Design review of the part built by this model. Coordinates are the model's own, in mm. Face numbers are marked on the shaded views. A direction names the side the tool comes from. Coordinates: 2 decimals unless noted, no trailing zeros. Write each loop counter-clockwise with the first axis right and the second up, starting at its lowest first coordinate (ties: lowest second). Pieces come first, ordered by that corner, then holes. Notation, with made-up numbers: (55.25, 60.5) - (85.25, 60.5) arc R15 cw to (85.25, 65.5) - close; hole circle Ø4 at (-6.5, 75.5). An arc over 180 degrees is marked (long way). Answer as CSV lines item,"result". Start each with the question number.
Q1. We need section B-B (x = 0). Write out the cut boundary in (y, z).
Q2. Mouldability with a two-part tool opening along X and no side actions: class the marked faces 3, 4 and 5 as pulls with the +X half, pulls with the -X half, needs draft (parallel to the pull), parting line crosses it, or undercut.
Q3. For line 1 along Z through (x, y) = (15, 17); line 2 along Z through (x, y) = (-4, 3); line 3 along X through (y, z) = (0, 27), list the stretches that pass through material, from the lowest coordinate up. Write a range as [from, to].
Q4. We need section C-C (z = 52). Write out the cut boundary in (x, y), plus the area to 3 significant figures.
Q5. Clearance check with flat-ended pins moving along their axes: pin 1 (10 mm diameter, centred on x = 7.5, y = 1, fed in from +Z); pin 2 (3 mm diameter, centred on x = 5.5, z = 44.5, fed in from -Y); pin 3 (5 mm diameter, centred on y = -0.5, z = 52.5, fed in from +X); pin 4 (3 mm diameter, centred on y = -0.5, z = 16.5, fed in from -X). State where each tip first meets the part, or that it passes through.
Q6. Machinability: for the marked faces 1 and 2, which of the approach directions +Z, -Z, +X, -X, +Y, -Y give a long, thin tool a straight path to every point of the face, cutting with its end or side? Answer none if there is none.
Q7. We need section A-A (y = 0). Write out the cut boundary in (x, z).
Q8. We need section D-D (z = 33). Write out the cut boundary in (x, y), plus the area to 3 significant figures.
from build123d import *

# Parameters (mm, degrees)
SKETCH1_R               = 7.5
BOSS_EXTRUDE1_DEPTH     = 56
SKETCH2_W               = 10
SKETCH2_H               = 16
CUT_EXTRUDE1_DEPTH      = 10
CUT_EXTRUDE4_DEPTH      = 57.995613866
CUT_EXTRUDE4_DEPTH_BACK = 57.995613866
CUT_EXTRUDE5_DEPTH      = 57.995613991
CUT_EXTRUDE5_DEPTH_BACK = 57.995613991
SKETCH4_R               = 1.5
FILLET1_R               = 0.1
SKETCH5_W               = 40
SKETCH5_H               = 40
BOSS_EXTRUDE2_DEPTH     = 5


with BuildPart() as part:
    # Sketch1 → Boss-Extrude1 (new body)
    with BuildSketch(Plane.XY):
        Circle(SKETCH1_R)
    extrude(amount=BOSS_EXTRUDE1_DEPTH)

    # Sketch2 → Cut-Extrude1 (cut)
    with BuildSketch(Plane.XY.offset(56)):
        Rectangle(SKETCH2_W, SKETCH2_H)
    extrude(amount=-CUT_EXTRUDE1_DEPTH, mode=Mode.SUBTRACT)

    # Sketch3 → Cut-Extrude4 (cut, two sides: drawn at the far end of the back side and taken through both)
    with BuildSketch(Plane(origin=(0, 0, 0), x_dir=(0, 0, -1), z_dir=(1, 0, 0)).offset(-CUT_EXTRUDE4_DEPTH_BACK)):
        with BuildLine():
            Line((-46, -114.267763227), (-46, -7.5))
            Line((-46, -7.5), (-46, -5.590169944))
            Line((-46, -5.590169944), (-52.952744721, -3.885047998))
            ThreePointArc((-52.952744721, -3.885047998), (-55.999999999, -0.000262165), (-52.952923855, 3.884664175))
            Line((-52.952923855, 3.884664175), (-46, 5.590169944))
            Line((-46, 5.590169944), (-46, 7.5))
            Line((-46, 7.5), (-46, 114.267763227))
            Line((-46, 114.267763227), (-259.535526454, 114.267763227))
            Line((-259.535526454, 114.267763227), (-259.535526454, -114.267763227))
            Line((-259.535526454, -114.267763227), (-46, -114.267763227))
        make_face()
    extrude(amount=CUT_EXTRUDE4_DEPTH + CUT_EXTRUDE4_DEPTH_BACK, mode=Mode.SUBTRACT)

    # Sketch4 → Cut-Extrude5 (cut, two sides: drawn at the far end of the back side and taken through both)
    with BuildSketch(Plane(origin=(0, 0, 0), x_dir=(0, 0, -1), z_dir=(1, 0, 0)).offset(-CUT_EXTRUDE5_DEPTH_BACK)):
        with Locations(Location((-52, -0.000169944, 0), (0, 0, 0.006491373))):
            Circle(SKETCH4_R)
    extrude(amount=CUT_EXTRUDE5_DEPTH + CUT_EXTRUDE5_DEPTH_BACK, mode=Mode.SUBTRACT)

    # Fillet1
    # the kernel refuses this fillet: 0.1 mm, written as the material it takes off along each edge
    with BuildSketch(Plane(origin=(0, 0, 46), x_dir=(0.6911452834399255, -0.7227158481580054, 0), z_dir=(0.7227158481580054, 0.6911452834399255, 0))) as fillet1_piece_1_section:
        with BuildLine():
            CenterArc((7.5 - FILLET1_R, FILLET1_R), FILLET1_R, 270, 90)
            Line((7.5 - FILLET1_R, 0), (7.5, 0))
            Line((7.5, 0), (7.5, FILLET1_R))
        make_face()
    fillet1_piece_1 = revolve(axis=Axis((0, 0, 46), (0, 0, -1)), revolution_arc=87.441672972, mode=Mode.PRIVATE)
    fillet1_piece_1 = split(fillet1_piece_1, bisect_by=Plane(origin=(5, -5.569278278, 45.983069625), z_dir=(-1, 0, 0)), keep=Keep.TOP, mode=Mode.PRIVATE)
    fillet1_piece_1 = split(fillet1_piece_1, bisect_by=Plane(origin=(-5, -5.569278278, 45.983069625), z_dir=(1, 0, 0)), keep=Keep.TOP, mode=Mode.PRIVATE)
    add(fillet1_piece_1, mode=Mode.SUBTRACT)
    with BuildSketch(Plane(origin=(0, 0, 46), x_dir=(-0.6911452834399255, 0.7227158481580054, 0), z_dir=(-0.7227158481580054, -0.6911452834399255, 0))) as fillet1_piece_2_section:
        with BuildLine():
            CenterArc((7.5 - FILLET1_R, FILLET1_R), FILLET1_R, 270, 90)
            Line((7.5 - FILLET1_R, 0), (7.5, 0))
            Line((7.5, 0), (7.5, FILLET1_R))
        make_face()
    fillet1_piece_2 = revolve(axis=Axis((0, 0, 46), (0, 0, -1)), revolution_arc=87.441672972, mode=Mode.PRIVATE)
    fillet1_piece_2 = split(fillet1_piece_2, bisect_by=Plane(origin=(5, 5.569279246, 45.98306893), z_dir=(-1, 0, 0)), keep=Keep.TOP, mode=Mode.PRIVATE)
    fillet1_piece_2 = split(fillet1_piece_2, bisect_by=Plane(origin=(-5, 5.569279246, 45.98306893), z_dir=(1, 0, 0)), keep=Keep.TOP, mode=Mode.PRIVATE)
    add(fillet1_piece_2, mode=Mode.SUBTRACT)

    # Sketch5 → Boss-Extrude2 (add)
    with BuildSketch(Plane(origin=(0, 0, 0), x_dir=(-1, 0, 0), z_dir=(0, 0, -1))):
        Rectangle(SKETCH5_W, SKETCH5_H)
    extrude(amount=BOSS_EXTRUDE2_DEPTH)


solid = part.part
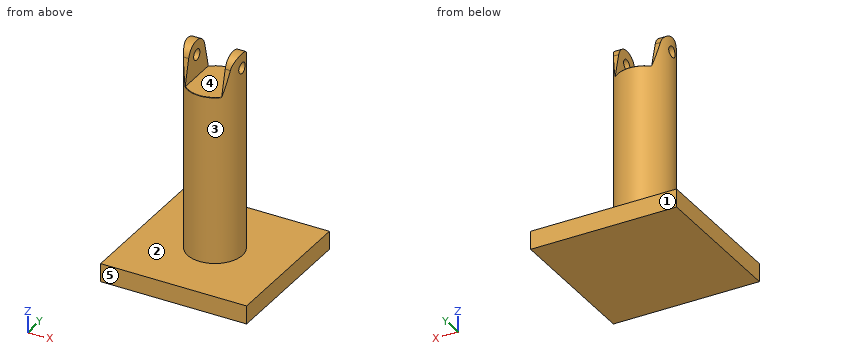
Results list:
1,outline,"(-20, -5) - (20, -5) - (20, 0) - (7.5, 0) - (7.5, 45.9) arc R0.1 ccw to (7.4, 46) - (-7.4, 46) arc R0.1 ccw to (-7.5, 45.9) - (-7.5, 0) - (-20, 0) - close"
2,face 3,"parting line crosses it"
2,face 4,"undercut"
2,face 5,"needs draft"
3,line 1,"z = [-5, 0]"
3,line 2,"z = [-5, 46]"
3,line 3,"x = [-7.5, 7.5]"
4,outline,"(-7.35, -1.5) arc R7.5 ccw to (-6.27, -4.12) - (-5, -4.12) - (-5, -1.5) - close; (-7.35, 1.5) - (-5, 1.5) - (-5, 4.12) - (-6.27, 4.12) arc R7.5 ccw to start; (5, -4.12) - (6.27, -4.12) arc R7.5 ccw to (7.35, -1.5) - (5, -1.5) - close; (5, 1.5) - (7.35, 1.5) arc R7.5 ccw to (6.27, 4.12) - (5, 4.12) - close"
4,area,"20.0 mm2"
5,pin 1,"stops at z = 56"
5,pin 2,"stops at y = -6.34"
5,pin 3,"stops at x = 7.5"
5,pin 4,"stops at x = -7.5"
6,face 1,"+Z, -Z, +X, -X, +Y"
6,face 2,"+Z"
7,outline,"(-20, -5) - (20, -5) - (20, 0) - (7.5, 0) - (7.5, 50.5) - (5, 50.5) - (5, 46) - (-5, 46) - (-5, 50.5) - (-7.5, 50.5) - (-7.5, 0) - (-20, 0) - close; (-7.5, 53.5) - (-5, 53.5) - (-5, 56) - (-7.5, 56) - close; (5, 53.5) - (7.5, 53.5) - (7.5, 56) - (5, 56) - close"
8,outline,"circle Ø15 at (0, 0)"
8,area,"177 mm2"
